```python
from build123d import *
from build123d.topology import SkipClean

# Parameters (mm, degrees)
SKETCH_1_R      = 5.02
SKETCH_1_R_2    = 0.93
EXTRUDE_1_DEPTH = 4.4
EXTRUDE_START   = 0.4
SKETCH_3_R      = 5.62
SKETCH_3_R_2    = 0.93
EXTRUDE_2_DEPTH = 0.4
CHAMFER_1_SIZE  = 0.5


with BuildPart() as part:
    # 草图1 → 凸台-拉伸1 (new body)
    with BuildSketch(Plane(origin=(0, 0, 0), x_dir=(1, 0, 0), z_dir=(0, 1, 0))):
        with Locations(Location((0, 0, 0), (0, 0, 270))):
            Circle(SKETCH_1_R)
        with Locations(Location((3.2, 0, 0), (0, 0, 270))):
            Circle(SKETCH_1_R_2, mode=Mode.SUBTRACT)
        with Locations(Location((-0.8, 0, 0), (0, 0, 90))):
            Circle(SKETCH_1_R_2, mode=Mode.SUBTRACT)
    extrude(amount=EXTRUDE_1_DEPTH)

    # 草图3 → 凸台-拉伸2 (add)
    with SkipClean():  # the faces are left unmerged after this step: merging them gives an invalid solid
        with BuildSketch(Plane.XZ.offset(EXTRUDE_START)):
            with Locations(Location((0, 0, 0), (0, 0, 270))):
                Circle(SKETCH_3_R)
            with Locations(Location((3.2, 0, 0), (0, 0, 270))):
                Circle(SKETCH_3_R_2, mode=Mode.SUBTRACT)
            with Locations(Location((-0.8, 0, 0), (0, 0, 270))):
                Circle(SKETCH_3_R_2, mode=Mode.SUBTRACT)
        extrude(amount=-EXTRUDE_2_DEPTH)

    # 倒角1
    # the kernel refuses this chamfer: 0.5 mm, written as the material it takes off along each edge
    with BuildSketch(Plane(origin=(3.2, -0.4, 0), x_dir=(0, 0, -1), z_dir=(-1, 0, 0))) as chamfer_1_piece_1:
        Polygon((0.93 + CHAMFER_1_SIZE, 0), (0.93, -CHAMFER_1_SIZE), (0.93, 0), align=None)
    revolve(axis=Axis((3.2, -0.4, 0), (0, -1, 0)), mode=Mode.SUBTRACT)
    with BuildSketch(Plane(origin=(-0.8, -0.4, 0), x_dir=(0, 0, -1), z_dir=(-1, 0, 0))) as chamfer_1_piece_2:
        Polygon((0.93 + CHAMFER_1_SIZE, 0), (0.93, -CHAMFER_1_SIZE), (0.93, 0), align=None)
    revolve(axis=Axis((-0.8, -0.4, 0), (0, -1, 0)), mode=Mode.SUBTRACT)
    with BuildSketch(Plane(origin=(0, 4.4, 0), x_dir=(0, 0, 1), z_dir=(-1, 0, 0))) as chamfer_1_piece_3:
        Polygon((5.02, -CHAMFER_1_SIZE), (5.02 - CHAMFER_1_SIZE, 0), (5.02, 0), align=None)
    revolve(axis=Axis((0, 4.4, 0), (0, 1, 0)), mode=Mode.SUBTRACT)
    with BuildSketch(Plane(origin=(3.2, 4.4, 0), x_dir=(0, 0, 1), z_dir=(-1, 0, 0))) as chamfer_1_piece_4:
        Polygon((0.93 + CHAMFER_1_SIZE, 0), (0.93, -CHAMFER_1_SIZE), (0.93, 0), align=None)
    revolve(axis=Axis((3.2, 4.4, 0), (0, 1, 0)), mode=Mode.SUBTRACT)
    with BuildSketch(Plane(origin=(-0.8, 4.4, 0), x_dir=(0, 0, -1), z_dir=(1, 0, 0))) as chamfer_1_piece_5:
        Polygon((0.93 + CHAMFER_1_SIZE, 0), (0.93, -CHAMFER_1_SIZE), (0.93, 0), align=None)
    revolve(axis=Axis((-0.8, 4.4, 0), (0, 1, 0)), mode=Mode.SUBTRACT)


solid = part.part
```
Part model, mm, in its own coordinate system. A direction names the side the tool comes from. Round coordinates to 2 decimals unless told otherwise and drop trailing zeros. Loops run counter-clockwise (first coordinate to the right, second up) from the corner with the lowest first, then second, coordinate; pieces in that order, holes last.
1. 3-axis set-ups, long thin cutter, end or side, ignore diameter. For faces 4 (the face through (1.508, 1.923, 4.788)), 5 (the face through (3.984, 1.973, 0.5)): which of +Z, -Z, +X, -X, +Y, -Y reach the whole face in a straight line?
Solutions:
face 4: +Y
face 5: +Y, -Y
2. Drill centre lines: line 1 along X through (y, z) = (2.8, 0); line 2 along X through (y, z) = (1.7, 0.75); line 3 along Z through (x, y) = (2.5, 3.5). Where is each one in solid material? Low to high.
Solutions:
line 1: x = -5.02 to -1.73, 0.13 to 2.27, 4.13 to 5.02
line 2: x = -4.96 to -1.35, -0.25 to 2.65, 3.75 to 4.96
line 3: z = -4.35 to -0.61, 0.61 to 4.35
3. Flat gauge pin, fed straight in: pin 1 (1.5 mm diameter, centred on x = 3.5, y = 1, fed in from -Z). Where does the tip first touch, or does it go through?
Solutions:
pin 1: stops at z = -4.2
4. Two-plate mould, pull along X, no slides. Class faces 1 (the face through (0.11, 1.97, 0.2)), 2 (the face through (-5.486, -0.203, 1.218)), 3 (the face through (1, 4.4, 0)): pulls with the +X half, pulls with the -X half, needs draft (parallel to the pull), parting line crosses it, or undercut.
Solutions:
face 1: undercut
face 2: parting line crosses it
face 3: needs draft
5. Slice it at A-A (z = 0). Give the cut face in (x, y) (3 decimals), and give its area (3 significant figures).
Solutions:
outline: (-5.62, -0.4) - (-2.23, -0.4) - (-1.73, 0.1) - (-1.73, 3.9) - (-2.23, 4.4) - (-4.52, 4.4) - (-5.02, 3.9) - (-5.02, 0) - (-5.62, 0) - close; (0.13, 0.1) - (0.63, -0.4) - (1.77, -0.4) - (2.27, 0.1) - (2.27, 3.9) - (1.77, 4.4) - (0.63, 4.4) - (0.13, 3.9) - close; (4.13, 0.1) - (4.63, -0.4) - (5.62, -0.4) - (5.62, 0) - (5.02, 0) - (5.02, 3.9) - (4.575, 4.345) - (4.13, 3.9) - close
area: 29.6 mm2
6. Slice it at B-B (y = 2.05). Give the cut face in (x, z), and give its area (3 significant figures).
Solutions:
outline: circle Ø10.04 at (0, 0); hole circle Ø1.86 at (-0.8, 0); hole circle Ø1.86 at (3.2, 0)
area: 73.7 mm2
